Geometry: see drawing. Coordinates: mm, zero at the bounding-box minimum. Coordinates: 2 decimals unless noted, no trailing zeros. Loops run counter-clockwise (first coordinate to the right, second up) from the corner with the lowest first, then second, coordinate; pieces in that order, holes last. Notation, with made-up numbers: M -18,-14.75 L 29,-14.75 A21 cw 29,-10.75 Z; hole C 50.5,8.25 d7. An arc over 180 degrees is marked long. One line per question, with ' | ' between items. Start each with the question number.
1. Ray query, probe 1 along X at (y, z) = (2.5, 2.85); probe 2 along Y at (x, z) = (5.08, 1.5) (1 decimal); probe 3 along Y at (x, z) = (21.08, 0.8) (3 decimals). Return the intervals inside material, ascending.
2. Pin query (flat end, axial travel): P1, Ø1.6, axis at y = 1.5, z = 2, coming from the +X side; P2, Ø1.4, axis at x = 21.08, y = 8.255, coming from the -Z side; P3, Ø1, axis at y = 1, z = 2, coming from the -X side; P4, Ø1.6, axis at x = 86.5, z = 2, coming from the -Y side (3 decimals). Return the tip coordinate at first contact, or that it passes through.
3. Section query B-B, the plane z = 0.75. State how many separate pieces and enclosed holes the cut face has, and give its area (3 significant figures).
4. Section query A-A, the plane x = 11.5. Output: boundary loops of the cut face in (y, z) (3 decimals), and give its area (3 significant figures).
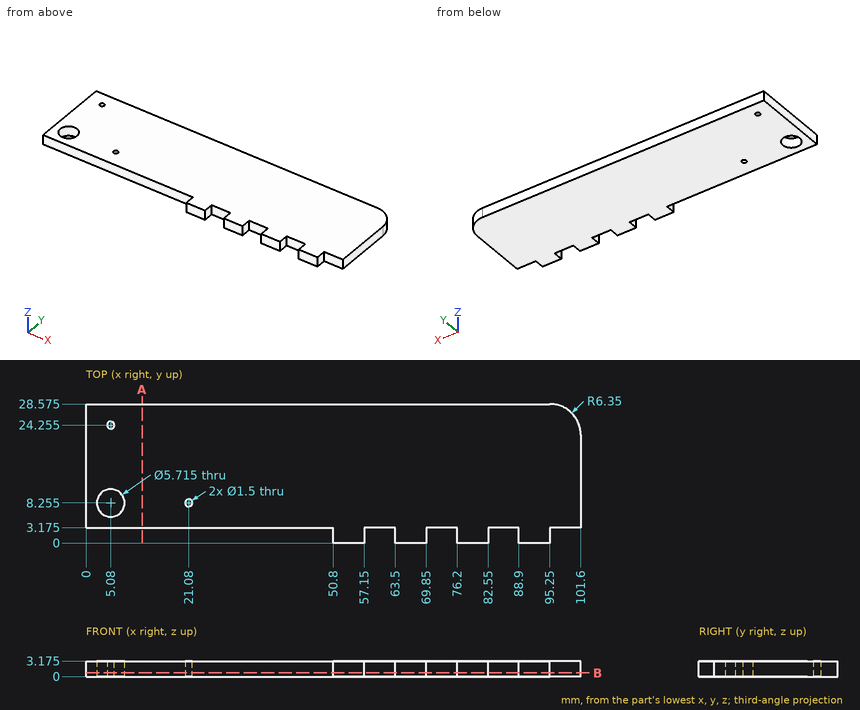
Taken from the geometry:
1) probe 1: 50.8 to 57.15, 63.5 to 69.85, 76.2 to 82.55, 88.9 to 95.25 | probe 2: 3.2 to 5.4, 11.1 to 23.5, 25 to 28.6 | probe 3: 3.175 to 7.505, 9.005 to 28.575
2) P1: x = 95.25 | P2: through | P3: x = 50.8 | P4: y = 3.175
3) separate pieces: 1 | enclosed holes: 3 | area: 2,620 mm^2
4) outline: M 3.175,0 L 28.575,0 L 28.575,3.175 L 3.175,3.175 Z | area: 80.6 mm^2
